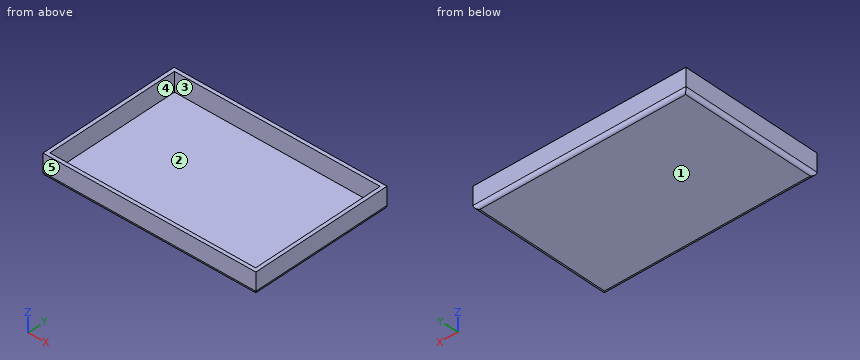
```python
from build123d import *

# Parameters (mm, degrees)
F0_W     = 300
F0_H     = 200
F0_W_2   = 295
F0_H_2   = 195
F0_W_3   = 290
F0_H_3   = 190
F1_DEPTH = 30
F2_DEPTH = 3
F3_DEPTH = 3
F4_R     = 5


with BuildPart() as f1:
    # F0 (on Top) → F1 (new body)
    with BuildSketch(Plane.XY):
        Rectangle(F0_W, F0_H)
        Rectangle(F0_W_2, F0_H_2, mode=Mode.SUBTRACT)
        Rectangle(F0_W_2, F0_H_2)
        Rectangle(F0_W_3, F0_H_3, mode=Mode.SUBTRACT)
    extrude(amount=F1_DEPTH)

    # F0 (on Top) → F2 (cut)
    with BuildSketch(Plane.XY):
        Rectangle(F0_W_2, F0_H_2)
        Rectangle(F0_W_3, F0_H_3, mode=Mode.SUBTRACT)
    extrude(amount=F2_DEPTH, mode=Mode.SUBTRACT)

    # F0 (on Top) → F3 (join)
    with BuildSketch(Plane.XY):
        Rectangle(F0_W_2, F0_H_2)
        Rectangle(F0_W_3, F0_H_3, mode=Mode.SUBTRACT)
        Rectangle(F0_W_3, F0_H_3)
    extrude(amount=F3_DEPTH)

    # F4
    f4_edges = [f1.edges().sort_by_distance(p)[0] for p in [
        (150, 0, 0),
        (0, 100, 0),
        (-150, 0, 0),
        (0, -100, 0),
    ]]
    fillet(f4_edges, radius=F4_R)


solid = f1.part
```
Here's how the part is built. I have some questions about the finished solid (model axes, mm). Face numbers are marked on the shaded views. A direction names the side the tool comes from. Round coordinates to 2 decimals unless told otherwise and drop trailing zeros. Write each loop counter-clockwise with the first axis right and the second up, starting at its lowest first coordinate (ties: lowest second). Pieces come first, ordered by that corner, then holes.
Q1. Will this pin go through, and if not, where does the flat tip stop? P1, Ø10, axis at x = 118.5, y = 75.5, coming from the +Z side.
Q2. If we section it at C-C on y = 39: Write out the boundary of the cut face in (x, z), plus the area to 3 significant figures.
Q3. Please list where these lines run through material, in increasing order: probe 1 along X at (y, z) = (-2, 7); probe 2 along Y at (x, z) = (-20, 12.75); probe 3 along Z at (x, y) = (-4, 69).
Q4. Which directions (+Z, -Z, +X, -X, +Y, -Y) give clear straight access to the entire face, cutting with the end or side of a thin tool? Please do the marked faces 4 and 5.
Q5. If we section it at B-B on x = -37: Write out the boundary of the cut face in (y, z).
Q6. If we mould it in two halves opening along X, with no side actions, what happens to the marked faces 1, 2 and 3? For each: +X half, -X half, draft (parallel to the pull), parting line (faces both ways), or undercut.
Q7. If we section it at A-A on z = 9.25: Write out the boundary of the cut face in (x, y).
Answer below:
1. P1: stops at z = 3
2. outline: (-150, 5) arc R5 ccw to (-145, 0) - (145, 0) arc R5 ccw to (150, 5) - (150, 30) - (145, 30) - (145, 3) - (-145, 3) - (-145, 30) - (-150, 30) - close
2. area: 1,160 mm2
3. probe 1: x = -150 to -145, 145 to 150
3. probe 2: y = -100 to -95, 95 to 100
3. probe 3: z = 0 to 3
4. face 4: +Z
4. face 5: +Z, -Z, +X, -X, -Y
5. outline: (-100, 5) arc R5 ccw to (-95, 0) - (95, 0) arc R5 ccw to (100, 5) - (100, 30) - (95, 30) - (95, 3) - (-95, 3) - (-95, 30) - (-100, 30) - close
6. face 1: draft
6. face 2: undercut
6. face 3: undercut
7. outline: (-150, -100) - (150, -100) - (150, 100) - (-150, 100) - close; hole (-145, -95) - (145, -95) - (145, 95) - (-145, 95) - close
